Design review of the part built by this model. Coordinates are the model's own, in mm. A direction names the side the tool comes from. Coordinates: 2 decimals unless noted, no trailing zeros. Loops run counter-clockwise (first coordinate to the right, second up) from the corner with the lowest first, then second, coordinate; pieces in that order, holes last. Notation, with made-up numbers: M 87,35 L 138,35 A13 cw 138,46 Z; hole C -20.5,10 d9. An arc over 180 degrees is marked long. Answer as a JSON object with one key per item and string values. Group by question number.
1. Insertion check: pin 1 (4 mm diameter, centred on x = -32, y = 34.5, fed in from +Z). The pin has a flat end and moves straight along its axis. Give the tip position at first contact, or say it passes through.
2. Consider section B-B (y = 135). State the section outline as (x, z) points.
3. To check wall thickness, follow probe 1 along Y at (x, z) = (-310, 12.25); probe 2 along X at (y, z) = (-95, 66.5); probe 3 along Y at (x, z) = (200, 230.5). State the ranges of each line that lie inside material, in increasing order.
4. Consider section D-D (y = 33). State the section outline as (x, z) points.
5. Consider section C-C (z = 80). State the section outline as (x, y) points.
6. Draft analysis for pull direction Z (two halves, no side actions). For faces 1 (the flat face through (363, 95, 166)), 2 (the flat face through (-30, 179, 335)), 3 (the flat face through (363, -95, 166)), 4 (the flat face through (5, 200, 165)), state which applies: +Z half, -Z half, draft (parallel to the pull), parting line (faces both ways), or undercut.
7. Consider section A-A (x = -310). State the section outline as (y, z) points, then the cut area to 3 significant figures.
8. Machinability: for faces 5 (the flat face through (-362, -1, 72.5)), 6 (the cylindrical face through (-286.154, 142.509, 12.675)), 7 (the flat face through (-350, -98, 178)), which of the approach directions +Z, -Z, +X, -X, +Y, -Y give a long, thin tool a straight path to every point of the face, cutting with its end or side? Answer none if there is none.
from build123d import *

# Parameters (mm, degrees)
F0_W     = 750
F0_H     = 400
F1_DEPTH = 25
F3_DEPTH = 310
F4_W     = 190
F4_H     = 190
F5_DEPTH = 750.001
F6_R     = 25
F7_DEPTH = 25.001


with BuildPart() as f1:
    # F0 (on Top) → F1 (new body)
    with BuildSketch(Plane.XY):
        Rectangle(F0_W, F0_H)
    extrude(amount=F1_DEPTH)

    # F2 (on face) → F3 (join)
    with BuildSketch(Plane.XY.offset(25)):
        Polygon((-350, -200), (-350, 175), (350, 175), (350, -200), (375, -200), (375, 200), (-375, 200), (-375, -200), align=None)
    extrude(amount=F3_DEPTH)

    # F4 (on face) → F5 (cut, through all)
    with BuildSketch(Plane.YZ.offset(375)):
        with Locations((0, 167.5)):
            Rectangle(F4_W, F4_H)
    extrude(amount=-F5_DEPTH, mode=Mode.SUBTRACT)

    # F6 (on face) → F7 (cut, through all)
    with BuildSketch(Plane.XY.offset(25)):
        with Locations((-310, 135)):
            Circle(F6_R)
    extrude(amount=-F7_DEPTH, mode=Mode.SUBTRACT)


solid = f1.part
Findings below:
{
 "1": {"pin 1": "stops at z = 25"},
 "2": {"outline": "M -375,0 L -335,0 L -335,25 L -350,25 L -350,335 L -375,335 Z; M -285,0 L 375,0 L 375,335 L 350,335 L 350,25 L -285,25 Z"},
 "3": {"probe 1": "y = -200 to 110, 160 to 200", "probe 2": "x = -375 to -350, 350 to 375", "probe 3": "y = 175 to 200"},
 "4": {"outline": "M -375,0 L 375,0 L 375,72.5 L 350,72.5 L 350,25 L -350,25 L -350,72.5 L -375,72.5 Z; M -375,262.5 L -350,262.5 L -350,335 L -375,335 Z; M 350,262.5 L 375,262.5 L 375,335 L 350,335 Z"},
 "5": {"outline": "M -375,-200 L -350,-200 L -350,-95 L -375,-95 Z; M -375,95 L -350,95 L -350,175 L 350,175 L 350,95 L 375,95 L 375,200 L -375,200 Z; M 350,-200 L 375,-200 L 375,-95 L 350,-95 Z"},
 "6": {"face 1": "undercut", "face 2": "+Z half", "face 3": "undercut", "face 4": "draft"},
 "7": {"outline": "M -200,0 L 110,0 L 110,25 L -200,25 Z; M 160,0 L 200,0 L 200,335 L 175,335 L 175,25 L 160,25 Z", "area": "16,500 mm^2"},
 "8": {"face 5": "+X, -X", "face 6": "+Z, -Z", "face 7": "+Z, -Y"}
}
